Autodesk Inventor part; units mm, degrees
ref_plane "YZ Plane" through (0, 0, 0) normal (1, 0, 0) x (0, 1, 0)
ref_plane "XZ Plane" through (0, 0, 0) normal (0, 1, 0) x (-1, 0, 0)
ref_plane "XY Plane" through (0, 0, 0) normal (0, 0, 1) x (1, 0, 0)
sketch "스케치1" plane through (0, 0, 0) normal (0, 1, 0) x (-1, 0, 0)
  line L0 (15, -12) -> (-15, -12)
  line L1 (-15, -12) -> (-15, 12)
  line L2 (-15, 12) -> (15, 12)
  line L3 (15, 12) -> (15, -12)
  line L4 (15, -12) -> (-15, 12) construction
  line L5 (-15, -12) -> (15, 12) construction
  line L6 (12.5, 9.5) -> (-12.5, 9.5)
  line L7 (-12.5, 9.5) -> (-12.5, -9.5)
  line L8 (-12.5, -9.5) -> (12.5, -9.5)
  line L9 (12.5, -9.5) -> (12.5, 9.5)
  line L10 (12.5, 9.5) -> (-12.5, -9.5) construction
  line L11 (-12.5, 9.5) -> (12.5, -9.5) construction
  circle A0 centre (12.5, -9.5) radius 1
  circle A1 centre (-12.5, -9.5) radius 1
  circle A2 centre (-12.5, 9.5) radius 1
  circle A3 centre (12.5, 9.5) radius 1
  point P0 (0, 0)
  dimension "d0" = 30
  dimension "d1" = 24
  dimension "d2" = 25
  dimension "d3" = 19
  dimension "d4" = 2
  dimension "d5" = 2
  dimension "d6" = 2
  dimension "d7" = 2
extrude "돌출1" add sketch "스케치1" along normal blind 1.2 contours L0 L1 L2 L3 | L6 A3 L9 A0 L8 A1 L7 A2
sketch "스케치2" plane through (0, 1.2, 0) normal (0, 1, 0) x (1, 0, 0)
  line L0 (-14, -7) -> (14, -7)
  line L1 (14, -7) -> (14, 7)
  line L2 (14, 7) -> (-14, 7)
  line L3 (-14, 7) -> (-14, -7)
  line L4 (-14, -7) -> (14, 7) construction
  line L5 (14, -7) -> (-14, 7) construction
  point P0 (0, 0)
  dimension "d10" = 28
  dimension "d11" = 14
extrude "돌출2" add sketch "스케치2" along normal blind 2
sketch "스케치3" plane through (0, 1.2, 0) normal (0, 1, 0) x (1, 0, 0)
  line L0 (15, -12) -> (15, 12)
  line L1 (15, 12) -> (-15, 12)
  circle A0 centre (-8.89, 10.56) radius 0.5
  circle A1 centre (-6.35, 10.56) radius 0.5
  circle A2 centre (-3.81, 10.56) radius 0.5
  circle A3 centre (-1.27, 10.56) radius 0.5
  circle A4 centre (1.27, 10.56) radius 0.5
  circle A5 centre (3.81, 10.56) radius 0.5
  circle A6 centre (6.35, 10.56) radius 0.5
  circle A7 centre (8.89, 10.56) radius 0.5
  point P0 (0, 0)
  dimension "d14" = 2.54
  dimension "d15" = 2.54
  dimension "d16" = 2.54
  dimension "d17" = 2.54
  dimension "d18" = 2.54
  dimension "d19" = 2.54
  dimension "d20" = 2.54
  dimension "d22" = 1.44
  dimension "d23" = 1
  dimension "d24" = 1
  dimension "d25" = 1
  dimension "d26" = 1
  dimension "d27" = 1
  dimension "d28" = 1
  dimension "d29" = 1
  dimension "d53" = 1
  dimension "d113" = 13.73
extrude "돌출3" add sketch "스케치3" along normal blind 2
chamfer "모따기1" distance 0.3 distance2 2 1 edges at (5.85, 3.2, -10.56) measured on face at (6.1668, 3.2, -10.6561)
chamfer "모따기2" distance 0.3 distance2 2 1 edges at (3.31, 3.2, -10.56) measured on face at (3.8691, 3.2, -10.4042)
chamfer "모따기3" distance 0.3 distance2 2 1 edges at (0.77, 3.2, -10.56) measured on face at (1.1007, 3.2, -10.7255)
chamfer "모따기4" distance 0.3 distance2 2 1 edges at (-1.77, 3.2, -10.56) measured on face at (-1.4393, 3.2, -10.7255)
chamfer "모따기5" distance 0.3 distance2 2 1 edges at (-4.31, 3.2, -10.56) measured on face at (-3.8038, 3.2, -10.4639)
chamfer "모따기6" distance 0.3 distance2 2 1 edges at (-6.85, 3.2, -10.56) measured on face at (-6.4319, 3.2, -10.5921)
chamfer "모따기7" distance 0.3 distance2 2 1 edges at (-9.39, 3.2, -10.56) measured on face at (-9.0639, 3.2, -10.4132)
chamfer "모따기8" distance 0.3 distance2 2 1 edges at (8.39, 3.2, -10.56) measured on face at (9.0549, 3.2, -10.6705)
sketch "스케치4" plane through (0, 0, 0) normal (0, -1, 0) x (1, 0, 0)
  circle A0 centre (6.35, -10.56) radius 0.5
  circle A1 centre (3.81, -10.56) radius 0.5
  circle A2 centre (1.27, -10.56) radius 0.5
  circle A3 centre (-1.27, -10.56) radius 0.5
  circle A4 centre (-3.81, -10.56) radius 0.5
  circle A5 centre (-6.35, -10.56) radius 0.5
  circle A6 centre (-8.89, -10.56) radius 0.5
  circle A7 centre (8.89, -10.56) radius 0.5
  line L0 (10.41, -11.83) -> (-10.41, -11.83)
  line L1 (-10.41, -11.83) -> (-10.41, -9.29)
  line L2 (-10.41, -9.29) -> (10.41, -9.29)
  line L3 (10.41, -9.29) -> (10.41, -11.83)
  point P0 (0, 0)
  dimension "d57" = 20.82
  dimension "d58" = 2.54
  dimension "d59" = 1.52
  dimension "d60" = 1.27
extrude "돌출4" add sketch "스케치4" along normal blind 2.5 contours A0 | A1 | A2 | A3 | A4 | A5 | A6 | A7 | L0 L1 L2 L3
sketch "스케치5" plane through (0, -2.5, 0) normal (0, -1, 0) x (1, 0, 0)
  circle A0 centre (8.89, -10.56) radius 0.5
  circle A1 centre (6.35, -10.56) radius 0.5
  circle A2 centre (3.81, -10.56) radius 0.5
  circle A3 centre (1.27, -10.56) radius 0.5
  circle A4 centre (-1.27, -10.56) radius 0.5
  circle A5 centre (-3.81, -10.56) radius 0.5
  circle A6 centre (-6.35, -10.56) radius 0.5
  circle A7 centre (-8.89, -10.56) radius 0.5
  line L0 (9.09, -10.86) -> (8.49, -10.86)
  line L1 (8.49, -10.86) -> (8.49, -10.26)
  line L2 (8.49, -10.26) -> (9.09, -10.26)
  line L3 (9.09, -10.26) -> (9.09, -10.86)
  line L4 (9.09, -10.86) -> (8.49, -10.26) construction
  line L5 (8.49, -10.86) -> (9.09, -10.26) construction
  line L6 (6.55, -10.86) -> (5.95, -10.86)
  line L7 (6.55, -10.26) -> (6.55, -10.86)
  line L8 (5.95, -10.26) -> (6.55, -10.26)
  line L9 (5.95, -10.86) -> (5.95, -10.26)
  line L10 (4.01, -10.86) -> (3.41, -10.86)
  line L11 (4.01, -10.26) -> (4.01, -10.86)
  line L12 (3.41, -10.26) -> (4.01, -10.26)
  line L13 (3.41, -10.86) -> (3.41, -10.26)
  line L14 (1.47, -10.86) -> (0.87, -10.86)
  line L15 (1.47, -10.26) -> (1.47, -10.86)
  line L16 (0.87, -10.26) -> (1.47, -10.26)
  line L17 (0.87, -10.86) -> (0.87, -10.26)
  line L18 (-1.07, -10.86) -> (-1.67, -10.86)
  line L19 (-1.07, -10.26) -> (-1.07, -10.86)
  line L20 (-1.67, -10.26) -> (-1.07, -10.26)
  line L21 (-1.67, -10.86) -> (-1.67, -10.26)
  line L22 (-3.61, -10.86) -> (-4.21, -10.86)
  line L23 (-3.61, -10.26) -> (-3.61, -10.86)
  line L24 (-4.21, -10.26) -> (-3.61, -10.26)
  line L25 (-4.21, -10.86) -> (-4.21, -10.26)
  line L26 (-6.15, -10.86) -> (-6.75, -10.86)
  line L27 (-6.15, -10.26) -> (-6.15, -10.86)
  line L28 (-6.75, -10.26) -> (-6.15, -10.26)
  line L29 (-6.75, -10.86) -> (-6.75, -10.26)
  line L30 (-8.69, -10.86) -> (-9.29, -10.86)
  line L31 (-8.69, -10.26) -> (-8.69, -10.86)
  line L32 (-9.29, -10.26) -> (-8.69, -10.26)
  line L33 (-9.29, -10.86) -> (-9.29, -10.26)
  point P0 (0, 0)
  point P1 (8.79, -10.56)
  point P2 (-1.27, -10.56)
  point P3 (-3.81, -10.56)
  point P4 (-6.35, -10.56)
  point P5 (-8.89, -10.56)
  dimension "d63" = 0.6
  dimension "d64" = 0.6
  dimension "d67" = 2.54
extrude "돌출5" add sketch "스케치5" along normal blind 6 contours L2 L3 L0 L1 | L8 L7 L6 L9 | L12 L11 L10 L13 | L16 L15 L14 L17 | L20 L19 L18 L21 | L24 L23 L22 L25 | L28 L27 L26 L29 | L32 L31 L30 L33
chamfer "모따기9" distance 0.15 angle 45 32 edges at (8.79, -8.5, -10.86) (8.49, -8.5, -10.56) (8.79, -8.5, -10.26) (9.09, -8.5, -10.56) (6.25, -8.5, -10.86) (6.55, -8.5, -10.56) (6.25, -8.5, -10.26) (5.95, -8.5, -10.56) (3.71, -8.5, -10.86) (3.41, -8.5, -10.56) (3.71, -8.5, -10.26) (4.01, -8.5, -10.56) (1.17, -8.5, -10.26) (0.87, -8.5, -10.56) (1.17, -8.5, -10.86) (1.47, -8.5, -10.56) (-1.37, -8.5, -10.86) (-1.07, -8.5, -10.56) (-1.37, -8.5, -10.26) (-1.67, -8.5, -10.56) (-3.91, -8.5, -10.86) (-3.61, -8.5, -10.56) (-3.91, -8.5, -10.26) (-4.21, -8.5, -10.56) (-6.15, -8.5, -10.56) (-6.45, -8.5, -10.86) (-6.75, -8.5, -10.56) (-6.45, -8.5, -10.26) (-8.99, -8.5, -10.86) (-8.69, -8.5, -10.56) (-8.99, -8.5, -10.26) (-9.29, -8.5, -10.56)
chamfer "모따기10" distance 1 angle 45 4 edges at (15, 0.6, -12) (15, 0.6, 12) (-15, 0.6, 12) (-15, 0.6, -12)
equation "\"d5\" = d4"
equation "\"d6\" = d4"
equation "\"d7\" = d4"
properties part number "SPI_Display_0.96inch"
Geometry: final body of the model. Coordinates: model frame, mm. A direction names the side the tool comes from. Round coordinates to 2 decimals unless told otherwise and drop trailing zeros. Write each loop counter-clockwise with the first axis right and the second up, starting at its lowest first coordinate (ties: lowest second). Pieces come first, ordered by that corner, then holes.
Item 1: Section query C-C (z = 6.25). Return loops of the section in (x, y), plus the area to 3 significant figures.
Item 2: Pin query (flat end, axial travel): P1, Ø0.7, axis at x = -6.5, y = -6, coming from the -Z side; P2, Ø6, axis at y = -3.5, z = -5.5, coming from the -X side; P3, Ø0.5, axis at x = -4, y = -5, coming from the +Z side; P4, Ø12, axis at x = -4, z = 1, coming from the -Y side. Return the tip coordinate at first contact, or that it passes through.
Item 3: Material intervals for L1, parallel to Z at x = 12.5, y = 0.8; L2, parallel to X at y = 0.55, z = 9.5; L3, parallel to X at y = 2.75, z = 0, sorted ascending.
Item 4: Set-up query: faces 4 (the face through (0, 1.2, 8)), 5 (the face through (0, 1, 12)), 6 (the face through (14, 2, 0)), 7 (the face through (-10.41, -1, -11)). Return all of +Z, -Z, +X, -X, +Y, -Y with unobstructed straight access to the full face (end or side cutting, diameter ignored); none if empty.
Item 5: Section query D-D (x = -8). Return loops of the section in (y, z), plus the area to 4 significant figures.
Item 6: Section query A-A (x = 12.5). Return loops of the section in (y, z), plus the area to 3 significant figures.
Item 7: Mould query, pull axis Z, two halves, no side actions, for faces 1 (the face through (1.194, 2.186, -10.904)), 2 (the face through (14.5, 0.6, -11.5)), 3 (the face through (14.5, 0.6, 11.5)). Classes: +Z half, -Z half, draft (parallel to the pull), parting line (faces both ways), or undercut.
Item 8: Section query B-B (y = -7). Give the number of separate pieces and of enclosed holes in the cut face, plus the area to 3 significant figures.
Completed:
1. outline: (-15, 0) - (15, 0) - (15, 1.2) - (14, 1.2) - (14, 3.2) - (-14, 3.2) - (-14, 1.2) - (-15, 1.2) - close
1. area: 92.0 mm2
2. P1: stops at z = -10.86
2. P2: passes through
2. P3: stops at z = -10.26
2. P4: stops at y = 0
3. L1: z = -12 to -10.5, -8.5 to 8.5, 10.5 to 12
3. L2: x = -15 to -13.5, -11.5 to 11.5, 13.5 to 15
3. L3: x = -14 to 14
4. face 4: +Y
4. face 5: +Z, +X, -X, +Y, -Y
4. face 6: +Z, -Z, +X, +Y
4. face 7: +Z, -Z, -X, -Y
5. outline: (-2.5, -11.83) - (0, -11.83) - (0, -12) - (1.2, -12) - (1.2, -7) - (3.2, -7) - (3.2, 7) - (1.2, 7) - (1.2, 12) - (0, 12) - (0, -9.29) - (-2.5, -9.29) - close
5. area: 63.15 mm2
6. outline: (0, -12) - (1.2, -12) - (1.2, -10.5) - (0, -10.5) - close; (0, -8.5) - (1.2, -8.5) - (1.2, -7) - (3.2, -7) - (3.2, 7) - (1.2, 7) - (1.2, 8.5) - (0, 8.5) - close; (0, 10.5) - (1.2, 10.5) - (1.2, 12) - (0, 12) - close
6. area: 52.0 mm2
7. face 1: undercut
7. face 2: -Z half
7. face 3: +Z half
8. separate pieces: 8
8. enclosed holes: 0
8. area: 2.88 mm2
